The drawing under review shows one solid part. Ordinate dimensions are in mm from its lowest x, y, z. A direction names the side the tool comes from. Coordinates: 2 decimals unless noted, no trailing zeros. Order: outer loops, then holes, each group sorted by start corner. A loop starts at its lowest first (then second) coordinate and runs counter-clockwise, first axis right, second up. Notation, with made-up numbers: (81.5, 64.5) -> (104.5, 64.5) arc R6 cw to (104.5, 68.5) -> close; hole circle Ø11 at (58.25, 13). An arc over 180 degrees is marked (long way). Use one line per item in the form item = value.
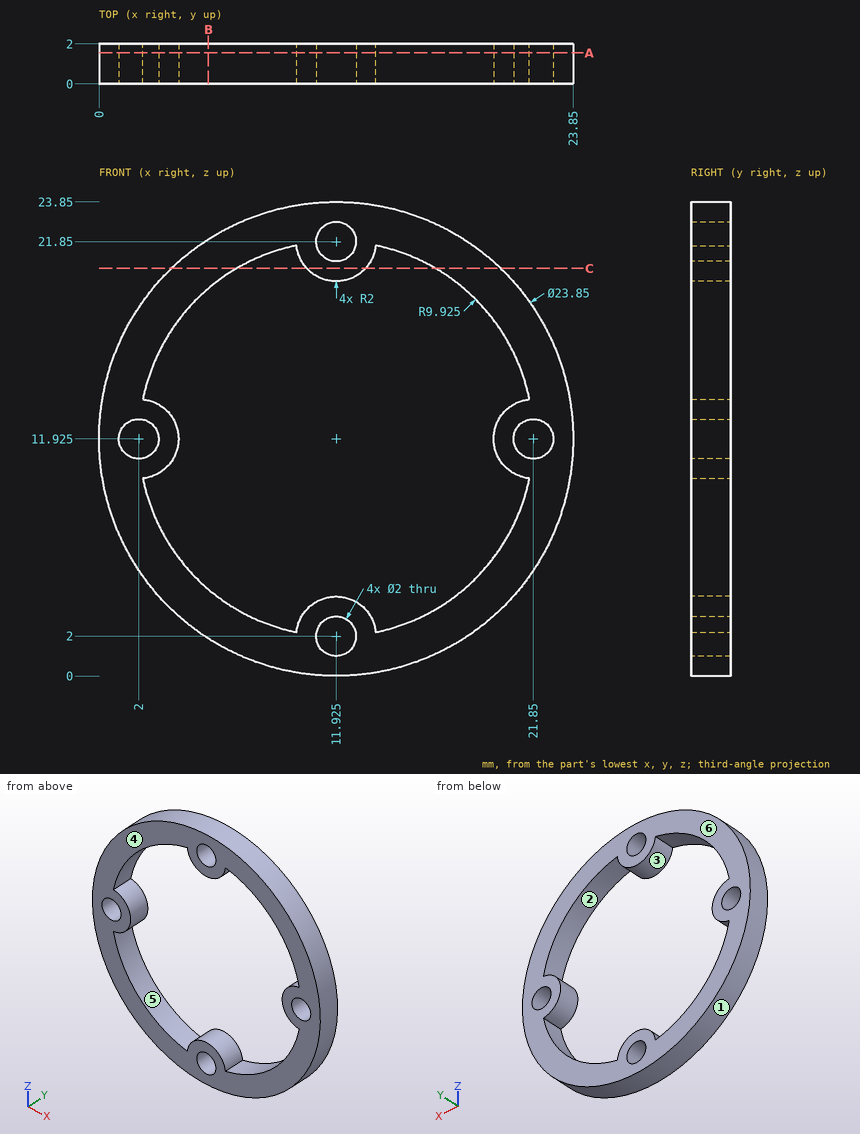
Item 1: Tool access review of the marked faces 5 and 6: name each direction out of +Z, -Z, +X, -X, +Y, -Y from which nothing blocks a thin tool from reaching the whole face with its end or side.
Results found:
face_5 = +Y, -Y
face_6 = +Z, -Z, +X, -X, +Y
Item 2: To check wall thickness, follow L1, parallel to Z at x = 12, y = 1.55; L2, parallel to X at y = 1.4, z = 20.75; L3, parallel to X at y = 0.6, z = 12.75. State the ranges of each line that lie inside material, in increasing order. Write a range as from..to.
Results found:
L1 = 0..1, 3..4, 19.85..20.85, 22.85..23.85
L2 = 3.9..7.38, 10.25..13.6, 16.47..19.95
L3 = 0.03..1.43, 2.57..3.82, 20.03..21.28, 22.42..23.82
Item 3: We need section C-C (z = 20.5). Write out the cut boundary in (x, y), plus the area to 3 significant figures.
Results found:
outline = (3.64, 0) -> (6.93, 0) -> (6.93, 2) -> (3.64, 2) -> close; (10.45, 0) -> (13.4, 0) -> (13.4, 2) -> (10.45, 2) -> close; (16.92, 0) -> (20.21, 0) -> (20.21, 2) -> (16.92, 2) -> close
area = 19.1 mm²
Item 4: Draft analysis for pull direction X (two halves, no side actions). For the marked faces 1, 2, 3 and 4, state which applies: released by +X, released by -X, zero draft, split by the parting line, or undercut.
Results found:
face_1 = split by the parting line
face_2 = undercut
face_3 = undercut
face_4 = zero draft
Item 5: We need section B-B (x = 5.5). Write out the cut boundary in (y, z).
Results found:
outline = (0, 1.88) -> (2, 1.88) -> (2, 4.36) -> (0, 4.36) -> close; (0, 19.49) -> (2, 19.49) -> (2, 21.97) -> (0, 21.97) -> close
Item 6: We need section A-A (y = 1.55). Write out the cut boundary in (x, z) (3 decimals).
Results found:
outline = circle Ø23.85 at (11.925, 11.925); hole circle Ø2 at (2, 11.925); hole (2.202, 9.935) arc R9.925 ccw to (9.935, 2.202) arc R2 cw to (13.915, 2.202) arc R9.925 ccw to (21.648, 9.935) arc R2 cw to (21.648, 13.915) arc R9.925 ccw to (13.915, 21.648) arc R2 cw to (9.935, 21.648) arc R9.925 ccw to (2.202, 13.915) arc R2 cw to start; hole circle Ø2 at (11.925, 2); hole circle Ø2 at (11.925, 21.85); hole circle Ø2 at (21.85, 11.925)
Item 7: Clearance check with a flat-ended pin moving along its axis: pin 1 (1 mm diameter, centred on y = 2, z = 18, fed in from -X). State where the tip first meets the part, or that it passes through.
Results found:
pin_1 = 1.38
